CAD build for the part. Positions are in the model's coordinates, mm. A direction names the side the tool comes from. Give positions to 0.01 mm unless a question says otherwise; leave off trailing zeros. Write each loop counter-clockwise with the first axis right and the second up, starting at its lowest first coordinate (ties: lowest second). Pieces come first, ordered by that corner, then holes. Notation, with made-up numbers: (88.5, 50.5) - (127.5, 50.5) arc R34 cw to (127.5, 80.5) - close; hole circle Ø2 at (-20, 39.25). An arc over 180 degrees is marked (long way). Put each result on its own line as item: value. Start each with the question number.
1. Cut at B-B on z = -37.5. List the corners of the cut face in (x, y).
2. Mould opens along Y. For faces 1 (the cylindrical face through (53.72, -39.37, -47.26)), 2 (the flat face through (52, 7, -37)), 3 (the cylindrical face through (39.626, 6.014, -33.745)) say: +Y half, -Y half, draft (parallel to the pull), parting line (faces both ways), or undercut.
3. Tool access for faces 4 (the flat face through (46, -85, -29)), 5 (the flat face through (52, -87, -37)): list every direction of +Z, -Z, +X, -X, +Y, -Y with a clear straight run to the whole face (end or side of a thin tool).
4. Cut at D-D on y = -67.5. List the corners of the cut face in (x, z), and give its area (3 significant figures).
5. Cut at C-C on x = 43.5. List the corners of the cut face in (y, z).
6. Drop flat-ended pins along their axis: pin 1 (2 mm diameter, centred on y = -51.5, z = -45.5, fed in from +X); pin 2 (3 mm diameter, centred on x = 54, y = -63.5, fed in from +Z); pin 3 (5 mm diameter, centred on x = 56, y = -48, fed in from -Z). Give the stop position or say it passes through.
7. Cut at A-A on z = -48.5. List the corners of the cut face in (x, y), and give its area (3 significant figures).
8. Wall check: line 1 (Y direction, x = 45.75, z = -29); line 2 (X direction, y = -53.5, z = -38); line 3 (Z direction, x = 55, y = -31.5). Give the ranges that are in metal, low to high.
Autodesk Inventor part; units mm, degrees
ref_plane "YZ Plane" through (0, 0, 0) normal (1, 0, 0) x (0, 1, 0)
ref_plane "XZ Plane" through (0, 0, 0) normal (0, 1, 0) x (-1, 0, 0)
ref_plane "XY Plane" through (0, 0, 0) normal (0, 0, 1) x (1, 0, 0)
ref_plane "Work Plane1" through (0, 0, 0) normal (0, 0, 1) x (1, 0, 0)
ref_plane "Work Plane2" through (0, 0, -37.5) normal (0, 0, 1) x (1, 0, 0)
sketch "Sketch1" plane through (0, 0, -37.5) normal (0, 0, 1) x (1, 0, 0)
  line L0 (41.5491, 5) -> (61.5491, 5)
  line L1 (41.5491, 5) -> (39.0491, 5)
  line L2 (39.0491, 5) -> (39.0491, 7)
  line L3 (39.0491, 7) -> (64.0491, 7)
  line L4 (64.0491, 7) -> (64.0491, 5)
  line L5 (64.0491, 5) -> (61.5491, 5)
  line L6 (61.5491, 5) -> (61.5491, -85)
  line L7 (61.5491, -85) -> (64.0491, -85)
  line L8 (64.0491, -85) -> (64.0491, -87)
  line L9 (64.0491, -87) -> (39.0491, -87)
  line L10 (39.0491, -87) -> (39.0491, -85)
  line L11 (39.0491, -85) -> (41.5491, -85)
  line L12 (41.5491, -85) -> (41.5491, 5)
  line L13 (51.5491, -97.5104) -> (51.5491, 34.0837)
  point P0 (0, 0)
  point P1 (51.5491, 7)
  point P2 (51.5491, -87)
  dimension "d1" = 2
  dimension "d5" = 90
  dimension "d12" = 25
  dimension "d13" = 2.5
revolve "Revolution1" add sketch "Sketch1" angle 360 about axis through (51.5491, -97.5104, -37.5) along (0, 1, 0) contours L1 L2 L3 L13 L0 | L0 L13 L9 L10 L11 L12
properties part number "nitR3"
Report:
1. outline: (39.05, -87) - (64.05, -87) - (64.05, -85) - (61.55, -85) - (61.55, 5) - (64.05, 5) - (64.05, 7) - (39.05, 7) - (39.05, 5) - (41.55, 5) - (41.55, -85) - (39.05, -85) - close
2. face 1: undercut
2. face 2: +Y half
2. face 3: draft
3. face 4: none
3. face 5: +Z, -Z, +X, -X, -Y
4. outline: circle Ø20 at (51.55, -37.5)
4. area: 314 mm²
5. outline: (-87, -47.06) - (-85, -47.06) - (-85, -43.43) - (5, -43.43) - (5, -47.06) - (7, -47.06) - (7, -27.94) - (5, -27.94) - (5, -31.57) - (-85, -31.57) - (-85, -27.94) - (-87, -27.94) - close
6. pin 1: stops at x = 58.69
6. pin 2: stops at z = -27.55
6. pin 3: stops at z = -47.31
7. outline: (45.61, -87) - (57.49, -87) - (57.49, -85) - (45.61, -85) - close; (45.61, 5) - (57.49, 5) - (57.49, 7) - (45.61, 7) - close
7. area: 47.5 mm²
8. line 1: y = -87 to -85, 5 to 7
8. line 2: x = 41.56 to 61.54
8. line 3: z = -46.89 to -28.11
